Geometry: see drawing. Coordinates: mm, zero at the bounding-box minimum. Coordinates: 2 decimals unless noted, no trailing zeros. Order: outer loops, then holes, each group sorted by start corner. A loop starts at its lowest first (then second) coordinate and runs counter-clockwise, first axis right, second up. Notation, with made-up numbers: M -18.5,62.5 L 37.5,62.5 A27 ccw 37.5,91.5 Z; hole C -13.75,30 d5. An arc over 180 degrees is marked long. Answer in a Markdown table with one row per item.
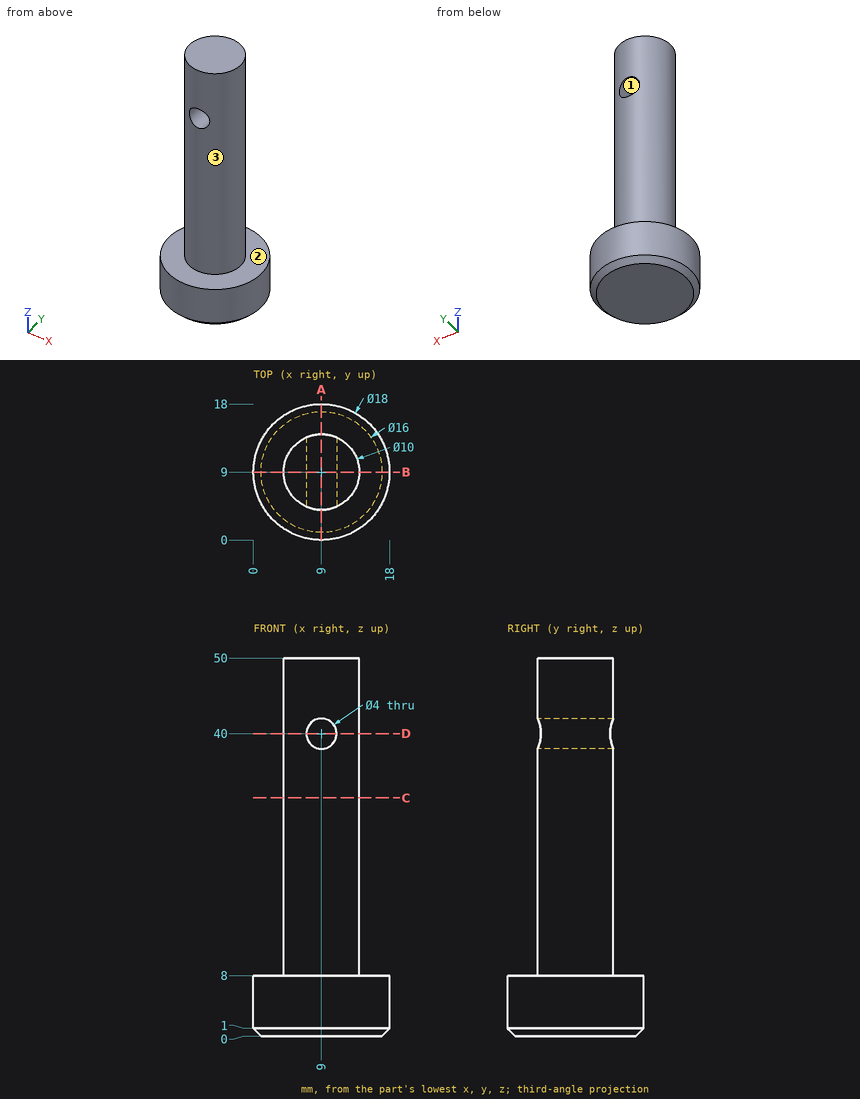
1) Cut plane B-B, the plane y = 9. Output: boundary loops of the cut face in (x, z).
Resolved:
| item | result |
|---|---|
| outline | M 0,1 L 1,0 L 17,0 L 18,1 L 18,8 L 14,8 L 14,50 L 4,50 L 4,8 L 0,8 Z; hole C 9,40 d4 |
2) Contact query for flat-ended pins moving along their axis: pin 1 (8 mm diameter, centred on x = 2.5, y = 5, fed in from -Z); pin 2 (5 mm diameter, centred on y = 14, z = 15.5, fed in from +X); pin 3 (1.5 mm diameter, centred on x = 7.5, y = 15.5, fed in from +Z); pin 4 (2 mm diameter, centred on x = 5, z = 19, fed in from +Y). Output: stop coordinate, or through.
Resolved:
| item | result |
|---|---|
| pin 1 | stops at z = 0 |
| pin 2 | stops at x = 13.33 |
| pin 3 | stops at z = 8 |
| pin 4 | stops at y = 13 |
3) Material intervals for probe 1 along Z at (x, y) = (9, 9.5); probe 2 along Z at (x, y) = (12.5, 13); probe 3 along Z at (x, y) = (8.5, 7.75), sorted ascending.
Resolved:
| item | result |
|---|---|
| probe 1 | z = 0 to 38, 42 to 50 |
| probe 2 | z = 0 to 8 |
| probe 3 | z = 0 to 38.06, 41.94 to 50 |
4) Mould query, pull axis X, two halves, no side actions, for the marked faces 1, 2 and 3. Classes: +X half, -X half, draft (parallel to the pull), parting line (faces both ways), or undercut.
Resolved:
| item | result |
|---|---|
| face 1 | undercut |
| face 2 | draft |
| face 3 | parting line |
5) Cut plane C-C, the plane z = 31.5. Output: boundary loops of the cut face in (x, y), and give its area (3 significant figures).
Resolved:
| item | result |
|---|---|
| outline | C 9,9 d10 |
| area | 78.5 mm2 |
6) Cut plane A-A, the plane x = 9. Output: boundary loops of the cut face in (y, z).
Resolved:
| item | result |
|---|---|
| outline | M 0,1 L 1,0 L 17,0 L 18,1 L 18,8 L 14,8 L 14,38 L 4,38 L 4,8 L 0,8 Z; M 4,42 L 14,42 L 14,50 L 4,50 Z |
7) Cut plane D-D, the plane z = 40. Output: boundary loops of the cut face in (x, y), and give its area (3 significant figures).
Resolved:
| item | result |
|---|---|
| outline | M 7,4.42 L 7,13.58 A5 ccw Z; M 11,4.42 A5 ccw 11,13.58 Z |
| area | 39.6 mm2 |
